Model file for the job. Use its own axes, mm. Give positions to 0.01 mm unless a question says otherwise; leave off trailing zeros. Loops run counter-clockwise (first coordinate to the right, second up) from the corner with the lowest first, then second, coordinate; pieces in that order, holes last. Notation, with made-up numbers: M 32.5,47.25 L 58.5,47.25 A10 ccw 58.5,64.25 Z; hole C -22,33 d2. An arc over 180 degrees is marked long. Answer in a Markdown table with one row per item.
Autodesk Inventor part; units mm, degrees
ref_plane "YZ Plane" through (0, 0, 0) normal (1, 0, 0) x (0, 1, 0)
ref_plane "XZ Plane" through (0, 0, 0) normal (0, 1, 0) x (-1, 0, 0)
ref_plane "XY Plane" through (0, 0, 0) normal (0, 0, 1) x (1, 0, 0)
sketch "Sketch1" plane through (0, 0, 0) normal (0, 1, 0) x (-1, 0, 0)
  line L0 (0, 0) -> (0, -2.5)
  line L1 (0, -2.5) -> (2.5, -5)
  line L2 (2.5, -5) -> (17.5, -5)
  line L3 (17.5, -5) -> (20, -2.5)
  line L4 (20, -2.5) -> (20, 0)
  line L5 (20, 0) -> (0, 0)
  point P0 (20, -1.25)
  dimension "d0" = 45
  dimension "d1" = 45
  dimension "d2" = 5
  dimension "d3" = 20
  dimension "d4" = 2.5
extrude "Extrusion1" add sketch "Sketch1" along normal blind 5
fillet "Fillet1" radius 2 2 edges at (-2.5, 2.5, -5) (-17.5, 2.5, -5)
equation "\"d2\" = glide_plate_height"
equation "\"d4\" = 0.5 * d2"
equation "\"d5\" = glide_plate_width"
equation "\"glide_plate_height\" = 5"
equation "\"glide_plate_length\" = 20"
equation "\"glide_plate_width\" = 5"
properties part number "steal_glide_plate"
Q1. Mould opens along X. For faces 1 (the face through (-20, 2, -1)), 2 (the face through (-10, 2, -5)), 3 (the face through (-2.553, 2.535, -4.844)) say: released by +X, released by -X, zero draft, split by the parting line, or undercut.
Reported:
| item | result |
|---|---|
| face 1 | released by -X |
| face 2 | zero draft |
| face 3 | released by +X |
Q2. Saw through at B-B (z = -3.45). Give the cut face in (x, y), and give its area (3 significant figures).
Reported:
| item | result |
|---|---|
| outline | M -19.05,0 L -0.95,0 L -0.95,5 L -19.05,5 Z |
| area | 90.5 mm² |
Q3. Saw through at C-C (x = -2.5). Give the cut face in (y, z).
Reported:
| item | result |
|---|---|
| outline | M 0,-4.82 L 5,-4.82 L 5,0 L 0,0 Z |
Q4. Saw through at A-A (y = 4.6). Give the cut face in (x, z), and give its area (3 significant figures).
Reported:
| item | result |
|---|---|
| outline | M -20,-2.5 L -18.09,-4.41 A2 ccw -16.67,-5 L -3.33,-5 A2 ccw -1.91,-4.41 L 0,-2.5 L 0,0 L -20,0 Z |
| area | 93.6 mm² |
Q5. Probe probe 1 along X at (y, z) = (4.6, -3.7); probe 2 along X at (y, z) = (2.6, -4.15); probe 3 along Z at (x, y) = (-2.5, 3.6). List the from-to ranges inside material, lowest first.
Reported:
| item | result |
|---|---|
| probe 1 | -18.8 to -1.2 |
| probe 2 | -18.35 to -1.65 |
| probe 3 | -4.82 to 0 |
